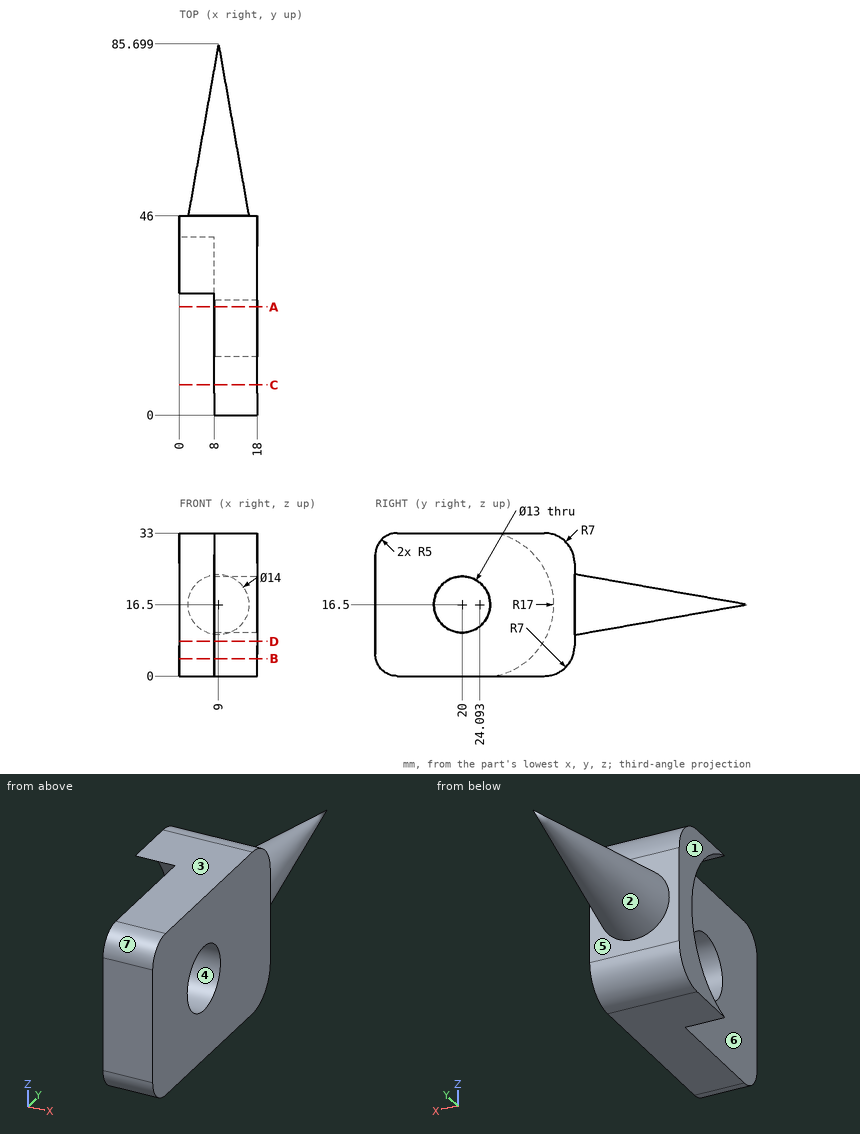
The figure shows three views and two pictorial views of one solid part (mm, origin at its lowest corner). Answer the questions. A direction names the side the tool comes from. Round coordinates to 2 decimals unless told otherwise and drop trailing zeros. Loops run counter-clockwise (first coordinate to the right, second up) from the corner with the lowest first, then second, coordinate; pieces in that order, holes last. Notation, with made-up numbers: M -30.75,66.5 L -12.75,66.5 A37 ccw -12.75,104.5 Z; hole C 71,-13 d2. An arc over 180 degrees is marked long. Use CSV: the item, a comma, the result in double quotes.
Q1. A tool of negligible diameter and unlimited length cuts with its end or side. For the marked faces 5, 6 and 7, from which of +Z, -Z, +X, -X, +Y, -Y can it reach the whole face along a straight path? Write none if from no direction.
Determined:
face 5,"+Y"
face 6,"-X, -Y"
face 7,"+Z, +X, -X, -Y"
Q2. Consider L1, parallel to Z at x = 13.75, y = 20; L2, parallel to X at y = 19, z = 24.5; L3, parallel to Y at x = 10.5, z = 7. Determine where each line is inside the solid, lowest interval first.
Determined:
L1,"0 to 10, 23 to 33"
L2,"8 to 18"
L3,"0 to 46"
Q3. Section C-C, the plane y = 7 is taken. Determine the outline of the cut face in (x, z).
Determined:
outline,"M 8,0 L 18,0 L 18,33 L 8,33 Z"
Q4. Section A-A, the plane y = 25 is taken. Determine the outline of the cut face in (x, z), then the cut area to 3 significant figures.
Determined:
outline,"M 8,0 L 18,0 L 18,12.35 L 8,12.35 Z; M 8,20.65 L 18,20.65 L 18,33 L 8,33 Z"
area,"247 mm2"
Q5. Section B-B, the plane z = 4 is taken. Determine the outline of the cut face in (x, y) (1 decimal), then the cut area to 3 significant figures.
Determined:
outline,"M 0,35.6 L 8,35.6 L 8,0.1 L 18,0.1 L 18,45.3 L 0,45.3 Z"
area,"530 mm2"
Q6. The mould has two halves that part along Z. Classify the marked faces 1, 2, 3 and 4: pulls with the +Z half, pulls with the -Z half, needs draft (parallel to the pull), parting line crosses it, or undercut.
Determined:
face 1,"needs draft"
face 2,"parting line crosses it"
face 3,"pulls with the +Z half"
face 4,"undercut"
Q7. Each of these flat-tipped pins is pushed along its axis until it touches: pin 1 (3 mm diameter, centred on x = 5.5, z = 24, fed in from -Y) (1 decimal); pin 2 (9 mm diameter, centred on x = 10, z = 17, fed in from +Y); pin 3 (10.5 mm diameter, centred on y = 20, z = 16.5, fed in from -X); pin 4 (6 mm diameter, centred on x = 14.5, z = 25.5, fed in from +Y). Where does it stop, or does it pass through?
Determined:
pin 1,"y = 38.5"
pin 2,"y = 85.7"
pin 3,"through"
pin 4,"y = 46"
Q8. Section D-D, the plane z = 8 is taken. Determine the outline of the cut face in (x, y) (1 decimal).
Determined:
outline,"M 0,38.8 L 8,38.8 L 8,0 L 18,0 L 18,46 L 0,46 Z"
